Read the model definition and answer for the solid it produces. Units are mm, in the model's axes. A direction names the side the tool comes from. Give positions to 0.01 mm unless a question says otherwise; leave off trailing zeros. Write each loop counter-clockwise with the first axis right and the second up, starting at its lowest first coordinate (ties: lowest second). Pieces come first, ordered by that corner, then holes. Notation, with made-up numbers: (-32, -5) -> (4, -5) arc R24 ccw to (4, 20) -> close; hole circle Ø10 at (-37.5, 49). An arc over 180 degrees is marked (long way). Use a Markdown table: item, result.
from build123d import *

# Parameters (mm, degrees)
ESQUISSE1_W             = 90
ESQUISSE1_H             = 32
BOSS_EXTRU_1_DEPTH      = 2
ESQUISSE2_W             = 90
ESQUISSE2_H             = 32
ESQUISSE2_W_2           = 86
ESQUISSE2_H_2           = 28
BOSS_EXTRU_3_DEPTH      = 45
ENL_V_MAT_EXTRU_1_REACH = 108.457
ESQUISSE3_W             = 6.41
ESQUISSE3_H             = 6.41
CONG_3_R                = 1
CHANFREIN8_SIZE         = 1
ESQUISSE7_W             = 65
ESQUISSE7_H             = 24
BOSS_EXTRU_8_DEPTH      = 7
CONG_11_R               = 3
CONG_12_R               = 3
ESQUISSE17_W            = 59
ESQUISSE17_H            = 5
ENL_V_MAT_EXTRU_6_DEPTH = 24
ESQUISSE20_W            = 46
ESQUISSE20_H            = 32
BOSS_EXTRU_10_DEPTH     = 20
ESQUISSE21_W            = 18
ESQUISSE21_H            = 28
ENL_V_MAT_EXTRU_7_DEPTH = 43
CONG_13_R               = 2
CONG_14_R               = 2
CONG_15_R               = 2
CONG_16_R               = 2
ESQUISSE22_W            = 3
ESQUISSE22_H            = 16
ENL_V_MAT_EXTRU_8_DEPTH = 2


with BuildPart() as part:
    # Esquisse1 → Boss.-Extru.1 (new body)
    with BuildSketch(Plane.XY):
        with Locations((45, 16)):
            Rectangle(ESQUISSE1_W, ESQUISSE1_H)
    extrude(amount=BOSS_EXTRU_1_DEPTH)

    # Esquisse2 → Boss.-Extru.3 (add)
    with BuildSketch(Plane.XY.offset(2)):
        with Locations((45, 16)):
            Rectangle(ESQUISSE2_W, ESQUISSE2_H)
        with Locations((45, 16)):
            Rectangle(ESQUISSE2_W_2, ESQUISSE2_H_2, mode=Mode.SUBTRACT)
    extrude(amount=BOSS_EXTRU_3_DEPTH)

    # Esquisse3 → Enlèv. mat.-Extru.1 (cut, up to next)
    with BuildSketch(Plane(origin=(90, 0, 0), x_dir=(0, 0, -1), z_dir=(1, 0, 0)), mode=Mode.PRIVATE) as enl_v_mat_extru_1_sk1:
        with Locations((-7.205, 20.445)):
            Rectangle(ESQUISSE3_W, ESQUISSE3_H)
    enl_v_mat_extru_1_tool1 = extrude(enl_v_mat_extru_1_sk1.sketch, amount=-ENL_V_MAT_EXTRU_1_REACH, mode=Mode.PRIVATE) & part.part
    add(enl_v_mat_extru_1_tool1.solids().sort_by_distance((90, 20.445, 7.205))[0], mode=Mode.SUBTRACT)

    # Congé3
    cong_3_edges = [part.edges().sort_by_distance(p)[0] for p in [
        (45, 2, 2),
        (88, 16, 2),
        (45, 30, 2),
        (2, 16, 2),
        (88, 2, 24.5),
        (88, 30, 24.5),
        (2, 30, 24.5),
        (2, 2, 24.5),
    ]]
    fillet(cong_3_edges, radius=CONG_3_R)

    # Chanfrein8
    chanfrein8_edges = [part.edges().sort_by_distance(p)[0] for p in [
        (45, 32, 0),
        (90, 16, 0),
        (45, 0, 0),
        (0, 16, 0),
    ]]
    chamfer(chanfrein8_edges, length=CHANFREIN8_SIZE)

    # Esquisse7 → Boss.-Extru.8 (add)
    with BuildSketch(Plane(origin=(0, 0, 0), x_dir=(-1, 0, 0), z_dir=(0, 0, -1))):
        with Locations((-37.5, 16)):
            Rectangle(ESQUISSE7_W, ESQUISSE7_H)
    extrude(amount=BOSS_EXTRU_8_DEPTH)

    # Congé11
    cong_11_edges = [part.edges().sort_by_distance(p)[0] for p in [
        (5, 16, -7),
    ]]
    fillet(cong_11_edges, radius=CONG_11_R)

    # Congé12
    cong_12_edges = [part.edges().sort_by_distance(p)[0] for p in [
        (70, 16, -7),
    ]]
    fillet(cong_12_edges, radius=CONG_12_R)

    # Esquisse17 → Enlèv. mat.-Extru.6 (cut)
    with BuildSketch(Plane(origin=(0, 28, 0), x_dir=(1, 0, 0), z_dir=(0, 1, 0))):
        with Locations((37.5, 2.5)):
            Rectangle(ESQUISSE17_W, ESQUISSE17_H)
    extrude(amount=-ENL_V_MAT_EXTRU_6_DEPTH, mode=Mode.SUBTRACT)

    # Esquisse20 → Boss.-Extru.10 (add)
    with BuildSketch(Plane.ZY):
        with Locations((24, 16)):
            Rectangle(ESQUISSE20_W, ESQUISSE20_H)
    extrude(amount=BOSS_EXTRU_10_DEPTH)

    # Esquisse21 → Enlèv. mat.-Extru.7 (cut)
    with BuildSketch(Plane.XY.offset(47)):
        with Locations((-9, 16)):
            Rectangle(ESQUISSE21_W, ESQUISSE21_H)
    extrude(amount=-ENL_V_MAT_EXTRU_7_DEPTH, mode=Mode.SUBTRACT)

    # Congé13
    cong_13_edges = [part.edges().sort_by_distance(p)[0] for p in [
        (0, 30, 25.5),
    ]]
    fillet(cong_13_edges, radius=CONG_13_R)

    # Congé14
    cong_14_edges = [part.edges().sort_by_distance(p)[0] for p in [
        (-18, 30, 25.5),
    ]]
    fillet(cong_14_edges, radius=CONG_14_R)

    # Congé15
    cong_15_edges = [part.edges().sort_by_distance(p)[0] for p in [
        (0, 2, 25.5),
    ]]
    fillet(cong_15_edges, radius=CONG_15_R)

    # Congé16
    cong_16_edges = [part.edges().sort_by_distance(p)[0] for p in [
        (-18, 2, 25.5),
    ]]
    fillet(cong_16_edges, radius=CONG_16_R)

    # Esquisse22 → Enlèv. mat.-Extru.8 (cut)
    with BuildSketch(Plane(origin=(2, 0, 0), x_dir=(0, 0, -1), z_dir=(1, 0, 0))):
        with Locations((-5.5, 16)):
            Rectangle(ESQUISSE22_W, ESQUISSE22_H)
    extrude(amount=-ENL_V_MAT_EXTRU_8_DEPTH, mode=Mode.SUBTRACT)


solid = part.part
Item 1: A cutting plane is placed at A-A (y = 11.5). Count the separate pieces of the cut face and the enclosed holes in it, then the cut area to 3 significant figures.
Return value:
| item | result |
|---|---|
| separate pieces | 2 |
| enclosed holes | 1 |
| area | 656 mm^2 |
Item 2: For a pull along Z with two mould halves and no side action, classify faces 5 (the face through (44, 30, 25)), 6 (the face through (69.1, 16.17, -6.14)), 7 (the face through (1, 8, 6)) as +Z half, -Z half, draft (parallel to the pull), parting line (faces both ways), or undercut.
Return value:
| item | result |
|---|---|
| face 5 | draft |
| face 6 | -Z half |
| face 7 | undercut |
Item 3: A cutting plane is placed at D-D (x = 76). Give the vertices of the cut face in (y, z).
Return value:
| item | result |
|---|---|
| outline | (0, 1) -> (1, 0) -> (31, 0) -> (32, 1) -> (32, 47) -> (30, 47) -> (30, 3) arc R1 cw to (29, 2) -> (3, 2) arc R1 cw to (2, 3) -> (2, 47) -> (0, 47) -> close |
Item 4: A cutting plane is placed at C-C (z = 41). Give the vertices of the cut face in (x, y), then the cut area to 3 significant figures.
Return value:
| item | result |
|---|---|
| outline | (-20, 0) -> (90, 0) -> (90, 32) -> (-20, 32) -> close; hole (-18, 4) arc R2 ccw to (-16, 2) -> (-2, 2) arc R2 ccw to (0, 4) -> (0, 28) arc R2 ccw to (-2, 30) -> (-16, 30) arc R2 ccw to (-18, 28) -> close; hole (2, 3) arc R1 ccw to (3, 2) -> (87, 2) arc R1 ccw to (88, 3) -> (88, 29) arc R1 ccw to (87, 30) -> (3, 30) arc R1 ccw to (2, 29) -> close |
| area | 612 mm^2 |
Item 5: A cutting plane is placed at B-B (x = 13.5). Give the vertices of the cut face in (y, z).
Return value:
| item | result |
|---|---|
| outline | (0, 1) -> (1, 0) -> (31, 0) -> (32, 1) -> (32, 47) -> (30, 47) -> (30, 3) arc R1 cw to (29, 2) -> (3, 2) arc R1 cw to (2, 3) -> (2, 47) -> (0, 47) -> close; (4, -7) -> (28, -7) -> (28, -5) -> (4, -5) -> close |
Item 6: Each of these flat-tipped pins is pushed along its axis until it touches: P1, Ø8, axis at x = 29, y = 14.5, coming from the +Z side; P2, Ø2.5, axis at y = 19, z = -3, coming from the +X side; P3, Ø3, axis at x = 3, y = 22, coming from the -Z side. Where does it stop, or does it pass through?
Return value:
| item | result |
|---|---|
| P1 | z = 2 |
| P2 | x = 70 |
| P3 | z = 0 |
Item 7: Straight lines are drawn through the part: line 1 along X through (y, z) = (7.5, 38.5); line 2 along Y through (x, z) = (36, 27.5); line 3 along Z through (x, y) = (35, 12). For each, find the intervals that lie inside material, in ascending order. Write a range as [from, to].
Return value:
| item | result |
|---|---|
| line 1 | [-20, -18], [0, 2], [88, 90] |
| line 2 | [0, 2], [30, 32] |
| line 3 | [-7, -5], [0, 2] |
Item 8: A tool of negligible diameter and unlimited length cuts with its end or side. For faces 1 (the face through (44, 2, 25)), 2 (the face through (89, 20, 4)), 3 (the face through (67, 16, -2)), 4 (the face through (1, 16, 7)), from which of +Z, -Z, +X, -X, +Y, -Y can it reach the whole face along a straight path? Write none if from no direction.
Return value:
| item | result |
|---|---|
| face 1 | +Z |
| face 2 | +X |
| face 3 | +Y, -Y |
| face 4 | none |
